Can you work these out from the drawing? Everything is in mm from the part's minimum corner. A direction names the side the tool comes from. Give positions to 0.01 mm unless a question says otherwise; leave off trailing zeros. Write each loop counter-clockwise with the first axis right and the second up, starting at its lowest first coordinate (ties: lowest second). Pieces come first, ordered by that corner, then holes. Notation, with made-up numbers: (44, -4) - (80, -4) arc R15 cw to (80, 21) - close; hole circle Ø4 at (40.5, 18). An arc over 180 degrees is marked (long way). Use a Markdown table: item, result.
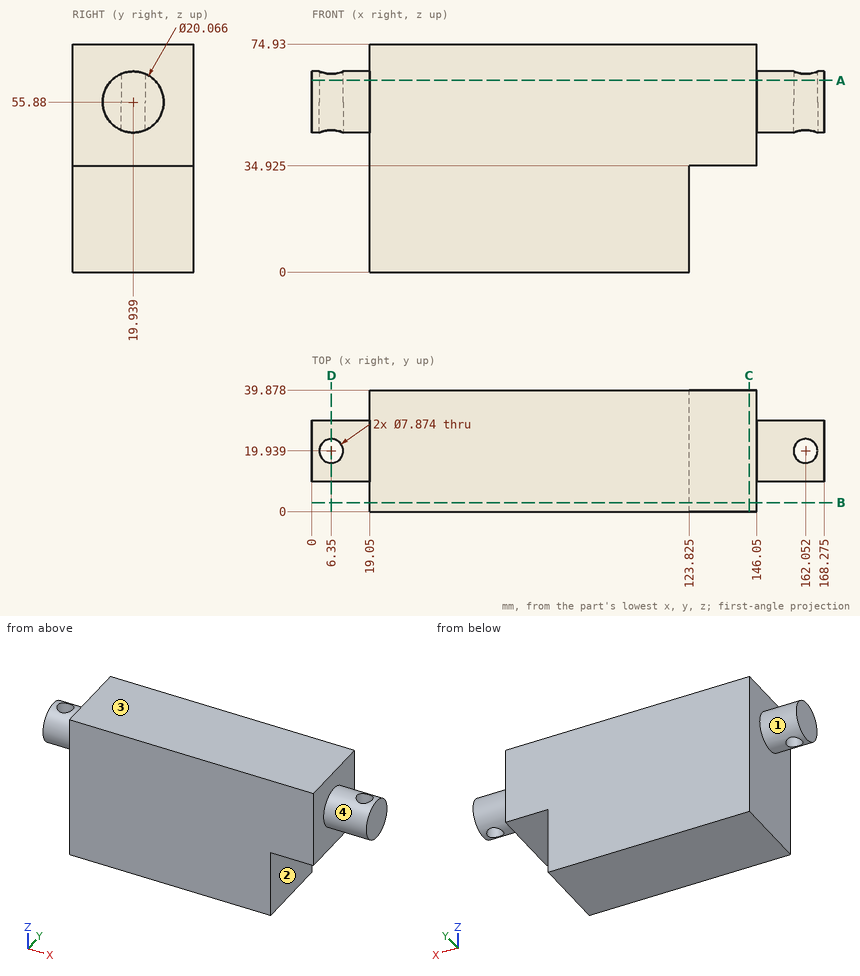
Item 1: For the marked faces 1, 2, 3 and 4, which set-ups out of +Z, -Z, +X, -X, +Y, -Y let a thin tool reach every point of the face, with its end or its side?
Values:
| item | result |
|---|---|
| face 1 | -X |
| face 2 | -Z, +X, +Y, -Y |
| face 3 | +Z, +X, -X, +Y, -Y |
| face 4 | +X |
Item 2: If we section it at B-B, the plane y = 3: Write out the boundary of the cut face in (x, z) (3 decimals), plus the area to 3 significant figures.
Values:
| item | result |
|---|---|
| outline | (19.05, 0) - (123.825, 0) - (123.825, 34.925) - (146.05, 34.925) - (146.05, 74.93) - (19.05, 74.93) - close |
| area | 8,740 mm2 |
Item 3: Will these pins go through, and if not, where does the flat tip stop? pin 1 Ø1.5 at (y, z) = (27.5, 9) entering from -X; pin 2 Ø7 at (x, y) = (162.052, 19.939) entering from +Z (3 decimals); pin 3 Ø18 at (x, y) = (134, 19.5) entering from -Z (3 decimals); pin 4 Ø1.5 at (y, z) = (28, 63.5) entering from +X.
Values:
| item | result |
|---|---|
| pin 1 | stops at x = 19.05 |
| pin 2 | passes through |
| pin 3 | stops at z = 34.925 |
| pin 4 | stops at x = 146.05 |
Item 4: If we section it at A-A, the plane z = 63: Write out the boundary of the cut face in (x, y) (3 decimals).
Values:
| item | result |
|---|---|
| outline | (0, 12.87) - (19.05, 12.87) - (19.05, 0) - (146.05, 0) - (146.05, 12.87) - (168.275, 12.87) - (168.275, 27.008) - (146.05, 27.008) - (146.05, 39.878) - (19.05, 39.878) - (19.05, 27.008) - (0, 27.008) - close; hole circle Ø7.874 at (6.35, 19.939); hole circle Ø7.874 at (162.052, 19.939) |
Item 5: I need wall thicknesses on line 1 along X through (y, z) = (3, 41); line 2 along X through (y, z) = (27, 21) (3 decimals); line 3 along Z through (x, y) = (155.5, 20.5). Which ranges of each line are inside material? Lowest first, please. Write a range as [from, to].
Values:
| item | result |
|---|---|
| line 1 | x = [19.05, 146.05] |
| line 2 | x = [19.05, 123.825] |
| line 3 | z = [45.86, 65.9] |
Item 6: If we section it at C-C, the plane x = 143.5: Write out the boundary of the cut face in (y, z) (3 decimals).
Values:
| item | result |
|---|---|
| outline | (0, 34.925) - (39.878, 34.925) - (39.878, 74.93) - (0, 74.93) - close |
Item 7: If we section it at D-D, the plane x = 6.35: Write out the boundary of the cut face in (y, z), plus the area to 3 significant figures.
Values:
| item | result |
|---|---|
| outline | (16, 46.65) - (16, 65.11) arc R10.03 ccw to start; (23.88, 46.65) arc R10.03 ccw to (23.88, 65.11) - close |
| area | 162 mm2 |
